Build history of the part. All positions in model axes, mm. Face numbers are marked on the shaded views. A direction names the side the tool comes from. Coordinates: 2 decimals unless noted, no trailing zeros. Write each loop counter-clockwise with the first axis right and the second up, starting at its lowest first coordinate (ties: lowest second). Pieces come first, ordered by that corner, then holes. Notation, with made-up numbers: (78, 73) -> (112, 73) arc R23 cw to (112, 87) -> close; hole circle Ø9 at (19.25, 22.5). An arc over 180 degrees is marked (long way). Write each question's results on one line, items separated by ' | '. Start each with the question number.
Q1. Saw through at C-C on x = 3.75. Give the cut face in (y, z).
Q2. Saw through at B-B on y = 4.25. Give the cut face in (x, z), and give its area (3 significant figures).
Q3. Saw through at A-A on z = 2.75. Give the cut face in (x, y).
Q4. Saw through at D-D on z = 1.5. Give the cut face in (x, y), and give its area (3 significant figures).
Q5. Tool access for the marked faces 5, 6 and 7: list every direction of +Z, -Z, +X, -X, +Y, -Y with a clear straight run to the whole face (end or side of a thin tool).
Q6. Two-plate mould, pull along X, no slides. Class the marked faces 1, 2, 3 and 4: released by +X, released by -X, zero draft, split by the parting line, or undercut.
Q7. Drill centre lines: line 1 (X direction, y = 0.45, z = 1); line 2 (X direction, y = 3.4, z = 0.25); line 3 (X direction, y = 1.1, z = 8.5). Where is each one in solid material? Low to high.
Q8. Drop a flat-ended pin along its axis: pin 1 Ø0.6 at (x, y) = (3.5, 3) entering from +Z. Give the stop position or say it passes through.
from build123d import *

# Parameters (mm, degrees)
BOSS_EXTRUDE1_DEPTH = 4.5


with BuildPart() as part:
    # Sketch1 → Boss-Extrude1 (new body)
    with BuildSketch(Plane(origin=(0, 0, 0), x_dir=(1, 0, 0), z_dir=(0, 1, 0))):
        with BuildLine():
            Line((-4.5, 0), (-4.5, -4.6))
            ThreePointArc((-4.5, -4.6), (-4.382842712, -4.882842712), (-4.1, -5))
            Line((-4.1, -5), (-2.901641857, -5))
            ThreePointArc((-2.901641857, -5), (-2.70339478, -4.947416315), (-2.557270511, -4.803490481))
            ThreePointArc((-2.557270511, -4.803490481), (-2.110791668, -4.620232906), (-1.812960087, -5))
            Line((-1.812960087, -5), (-1.75, -8.606980963))
            ThreePointArc((-1.75, -8.606980963), (-1.630424628, -8.88530018), (-1.350060922, -9))
            Line((-1.350060922, -9), (1.350060922, -9))
            ThreePointArc((1.350060922, -9), (1.630424628, -8.88530018), (1.75, -8.606980963))
            Line((1.75, -8.606980963), (1.812960087, -5))
            ThreePointArc((1.812960087, -5), (2.110791668, -4.620232906), (2.557270511, -4.803490481))
            ThreePointArc((2.557270511, -4.803490481), (2.70339478, -4.947416315), (2.901641857, -5))
            Line((2.901641857, -5), (4.1, -5))
            ThreePointArc((4.1, -5), (4.382842712, -4.882842712), (4.5, -4.6))
            Line((4.5, -4.6), (4.5, 0))
            ThreePointArc((4.5, 0), (3.75, 0.75), (3, 0))
            ThreePointArc((3, 0), (0, -3), (-3, 0))
            ThreePointArc((-3, 0), (-3.75, 0.75), (-4.5, 0))
        make_face()
    extrude(amount=BOSS_EXTRUDE1_DEPTH)


solid = part.part
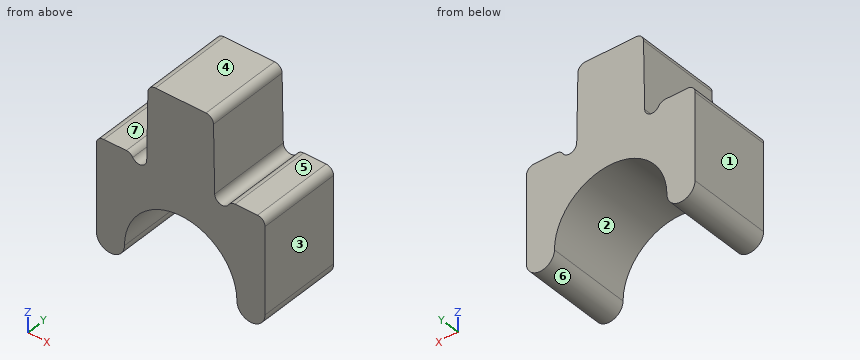
Returned:
1) outline: (0, -0.75) -> (4.5, -0.75) -> (4.5, 5) -> (0, 5) -> close
2) outline: (-4.5, 0) arc R0.75 ccw to (-3, 0) arc R3 cw to (3, 0) arc R0.75 ccw to (4.5, 0) -> (4.5, 4.6) arc R0.4 ccw to (4.1, 5) -> (2.9, 5) arc R0.4 ccw to (2.56, 4.8) arc R0.4 cw to (1.81, 5) -> (1.75, 8.61) arc R0.4 ccw to (1.35, 9) -> (-1.35, 9) arc R0.4 ccw to (-1.75, 8.61) -> (-1.81, 5) arc R0.4 cw to (-2.56, 4.8) arc R0.4 ccw to (-2.9, 5) -> (-4.1, 5) arc R0.4 ccw to (-4.5, 4.6) -> close | area: 46.2 mm2
3) outline: (-4.5, 0) -> (-1.2, 0) -> (-1.2, 4.5) -> (-4.5, 4.5) -> close; (1.2, 0) -> (4.5, 0) -> (4.5, 4.5) -> (1.2, 4.5) -> close
4) outline: (-4.5, 0) -> (-2.6, 0) -> (-2.6, 4.5) -> (-4.5, 4.5) -> close; (2.6, 0) -> (4.5, 0) -> (4.5, 4.5) -> (2.6, 4.5) -> close | area: 17.1 mm2
5) face 5: +Z, +X, +Y, -Y | face 6: -Z, +Y, -Y | face 7: +Z, -X, +Y, -Y
6) face 1: released by -X | face 2: undercut | face 3: released by +X | face 4: zero draft
7) line 1: x = -4.5 to -2.83, 2.83 to 4.5 | line 2: x = -4.5 to -2.99, 2.99 to 4.5 | line 3: x = -1.75 to 1.75
8) pin 1: stops at z = 5
